Could you check a few things on this model? Use its own coordinates, in mm. Coordinates: 2 decimals unless noted, no trailing zeros. Loops run counter-clockwise (first coordinate to the right, second up) from the corner with the lowest first, then second, coordinate; pieces in that order, holes last. Notation, with made-up numbers: (-10, -40) -> (13, -40) arc R25 ccw to (13, -3) -> close; hole circle Ø2 at (17.5, 24.5). An arc over 180 degrees is marked (long way). One line per question, with ' | ' between items.
from build123d import *

# Parameters (mm, degrees)
SKETCH_1_R      = 2
EXTRUDE_1_DEPTH = 3


with BuildPart() as part:
    # 草图1 → 凸台-拉伸1 (new body)
    with BuildSketch(Plane.XZ.offset(3)):
        with BuildLine():
            Line((162, -82.2), (162, 82.2))
            ThreePointArc((162, 82.2), (160.887005769, 84.887005769), (158.2, 86))
            Line((158.2, 86), (-158.2, 86))
            ThreePointArc((-158.2, 86), (-160.887005769, 84.887005769), (-162, 82.2))
            Line((-162, 82.2), (-162, -82.2))
            ThreePointArc((-162, -82.2), (-160.887005769, -84.887005769), (-158.2, -86))
            Line((-158.2, -86), (158.2, -86))
            ThreePointArc((158.2, -86), (160.887005769, -84.887005769), (162, -82.2))
        make_face()
        with Locations((-144.95, 66.75)):
            Circle(SKETCH_1_R, mode=Mode.SUBTRACT)
        with Locations((-144.95, -66.75)):
            Circle(SKETCH_1_R, mode=Mode.SUBTRACT)
        with Locations((144.95, -66.75)):
            Circle(SKETCH_1_R, mode=Mode.SUBTRACT)
        with Locations((144.95, 66.75)):
            Circle(SKETCH_1_R, mode=Mode.SUBTRACT)
        with Locations((157, 45)):
            Circle(SKETCH_1_R, mode=Mode.SUBTRACT)
        with Locations((157, -45)):
            Circle(SKETCH_1_R, mode=Mode.SUBTRACT)
        with Locations((125, -81)):
            Circle(SKETCH_1_R, mode=Mode.SUBTRACT)
        with Locations((-125, -81)):
            Circle(SKETCH_1_R, mode=Mode.SUBTRACT)
        with Locations((-157, -45)):
            Circle(SKETCH_1_R, mode=Mode.SUBTRACT)
        with Locations((-157, 45)):
            Circle(SKETCH_1_R, mode=Mode.SUBTRACT)
        with Locations((125, 81)):
            Circle(SKETCH_1_R, mode=Mode.SUBTRACT)
        with Locations((-125, 81)):
            Circle(SKETCH_1_R, mode=Mode.SUBTRACT)
        with BuildLine():
            Line((2, 58), (2, 56))
            ThreePointArc((2, 56), (2.305807419, 54.466070022), (3.176470588, 53.166683629))
            ThreePointArc((3.176470588, 53.166683629), (0, 45.479202711), (-3.176470588, 53.166683629))
            ThreePointArc((-3.176470588, 53.166683629), (-2.305807419, 54.466070022), (-2, 56))
            Line((-2, 56), (-2, 58))
            ThreePointArc((-2, 58), (0, 60), (2, 58))
        make_face(mode=Mode.SUBTRACT)
        with BuildLine():
            Line((25, 15), (25, -15))
            ThreePointArc((25, -15), (23.535533906, -18.535533906), (20, -20))
            Line((20, -20), (-20, -20))
            ThreePointArc((-20, -20), (-23.535533906, -18.535533906), (-25, -15))
            Line((-25, -15), (-25, 15))
            ThreePointArc((-25, 15), (-23.535533906, 18.535533906), (-20, 20))
            Line((-20, 20), (20, 20))
            ThreePointArc((20, 20), (23.535533906, 18.535533906), (25, 15))
        make_face(mode=Mode.SUBTRACT)
    extrude(amount=-EXTRUDE_1_DEPTH)


solid = part.part
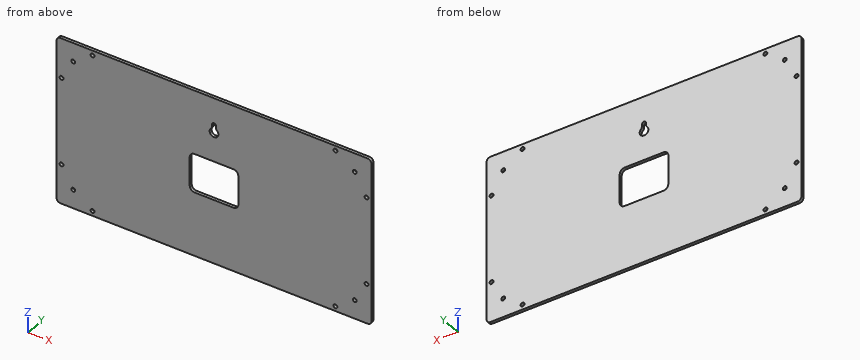
1) If we section it at A-A on z = -2: Please give me the cut outline in (x, y), and give its area (3 significant figures).
Data:
outline: (-162, -3) -> (-25, -3) -> (-25, 0) -> (-162, 0) -> close; (25, -3) -> (162, -3) -> (162, 0) -> (25, 0) -> close | area: 822 mm²
2) I need wall thicknesses on line 1 along Z through (x, y) = (0, -2.3); line 2 along Z through (x, y) = (-125, -2.2); line 3 along X through (y, z) = (-2.6, 10.5). Which ranges of each line are inside material? Lowest first, please. Write a range as from..to.
Data:
line 1: -86..-20, 20..45.48, 60..86 | line 2: -86..-83, -79..79, 83..86 | line 3: -162..-25, 25..162
3) If we section it at B-B on y = -0.6: Give the number of separate pieces and of enclosed holes in the cut face, and give its area (3 significant figures).
Data:
separate pieces: 1 | enclosed holes: 14 | area: 53,500 mm²
4) I'm going to push a flat-ended pin straight in: pin 1 Ø3.5 at (x, z) = (-144.95, 66.75) entering from +Y. Where does the tip first touch, or does it pass through?
Data:
pin 1: through
